Source: CAD feature listing. Evaluate the final solid. Frame: model axes, mm. Give positions to 0.01 mm unless a question says otherwise; leave off trailing zeros. Loops run counter-clockwise (first coordinate to the right, second up) from the corner with the lowest first, then second, coordinate; pieces in that order, holes last. Notation, with made-up numbers: M 77,30.25 L 125,30.25 A17 ccw 125,57.25 Z; hole C -14.5,34 d5. An arc over 180 degrees is marked long. Answer in a Markdown table with one row per item.
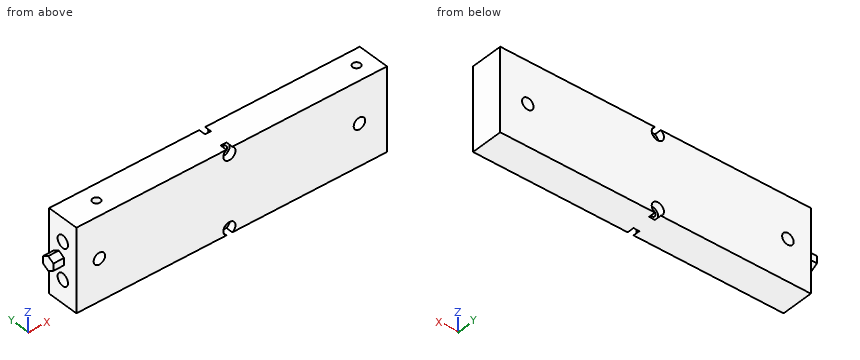
```python
from build123d import *

# Parameters (mm, degrees)
SKETCH_1_W          = 203
SKETCH_1_H          = 54
EXTRUDE_1_DEPTH     = 21
SKETCH_2_R          = 4
CUT_EXTRUDE_1_DEPTH = 150
SKETCH_3_R          = 2.25
CUT_EXTRUDE_2_DEPTH = 212.106608139
SKETCH_4_R          = 4
CUT_EXTRUDE_3_DEPTH = 4.5
SKETCH_5_R          = 3.75
CUT_EXTRUDE_4_DEPTH = 7.2
SKETCH_6_R          = 2.5
CUT_EXTRUDE_5_DEPTH = 5
EXTRUDE_2_DEPTH     = 7


with BuildPart() as part:
    # 草图1 → 凸台-拉伸1 (new body)
    with BuildSketch(Plane(origin=(0, 0, 0), x_dir=(1, 0, 0), z_dir=(0, 1, 0))):
        with Locations((101.5, 27)):
            Rectangle(SKETCH_1_W, SKETCH_1_H)
    extrude(amount=EXTRUDE_1_DEPTH)

    # 草图2 → 切除-拉伸1 (cut)
    with BuildSketch(Plane.ZY):
        with Locations((-15, 10.5)):
            Circle(SKETCH_2_R)
        with Locations(Location((-39, 10.5, 0), (0, 0, 180))):
            Circle(SKETCH_2_R)
    extrude(amount=-CUT_EXTRUDE_1_DEPTH, mode=Mode.SUBTRACT)

    # 草图3 → 切除-拉伸2 (cut, through all)
    with BuildSketch(Plane(origin=(0, 21, 0), x_dir=(1, 0, 0), z_dir=(0, 1, 0))):
        with Locations(Location((100, 3.5, 0), (0, 0, 270))):
            Circle(SKETCH_3_R)
        with Locations(Location((100, 50.5, 0), (0, 0, 270))):
            Circle(SKETCH_3_R)
        with Locations(Location((15, 27, 0), (0, 0, 270))):
            Circle(SKETCH_3_R)
        with Locations(Location((185, 27, 0), (0, 0, 270))):
            Circle(SKETCH_3_R)
    extrude(amount=-CUT_EXTRUDE_2_DEPTH, mode=Mode.SUBTRACT)

    # 草图4 → 切除-拉伸3 (cut)
    with BuildSketch(Plane(origin=(0, 21, 0), x_dir=(1, 0, 0), z_dir=(0, 1, 0))):
        with Locations((100, 50.5)):
            Circle(SKETCH_4_R)
        with Locations((100, 3.5)):
            Circle(SKETCH_4_R)
    cut_extrude_3 = extrude(amount=-CUT_EXTRUDE_3_DEPTH, mode=Mode.SUBTRACT)

    # 草图5 → 切除-拉伸4 (cut)
    with BuildSketch(Plane(origin=(0, 21, 0), x_dir=(1, 0, 0), z_dir=(0, 1, 0))):
        with Locations(Location((185, 27, 0), (0, 0, 270))):
            Circle(SKETCH_5_R)
        with Locations(Location((15, 27, 0), (0, 0, 270))):
            Circle(SKETCH_5_R)
    cut_extrude_4 = extrude(amount=-CUT_EXTRUDE_4_DEPTH, mode=Mode.SUBTRACT)

    # 镜向1: 切除-拉伸3, 切除-拉伸4 across plane
    add(cut_extrude_3.mirror(Plane(origin=(0, 10.5, 0), x_dir=(0, 0, 1), z_dir=(0, -1, 0))), mode=Mode.SUBTRACT)
    add(cut_extrude_4.mirror(Plane(origin=(0, 10.5, 0), x_dir=(0, 0, 1), z_dir=(0, -1, 0))), mode=Mode.SUBTRACT)

    # 草图6 → 切除-拉伸5 (cut)
    with BuildSketch(Plane.XY):
        with Locations((22, 10.5)):
            Circle(SKETCH_6_R)
        with Locations((192, 10.5)):
            Circle(SKETCH_6_R)
    extrude(amount=-CUT_EXTRUDE_5_DEPTH, mode=Mode.SUBTRACT)

    # 草图7 → 凸台-拉伸2 (add)
    with BuildSketch(Plane.ZY):
        Polygon((-24.690598923, 17.5), (-29.309401077, 17.5), (-31.618802154, 13.5), (-29.309401077, 9.5), (-24.690598923, 9.5), (-22.381197846, 13.5), align=None)
    extrude(amount=EXTRUDE_2_DEPTH)


solid = part.part
```
1) Section C-C, the plane z = -39. Return loops of the section in (x, y), then the cut area to 3 significant figures.
Reply:
| item | result |
|---|---|
| outline | M 0,0 L 203,0 L 203,21 L 0,21 L 0,14.5 L 150,14.5 L 150,6.5 L 0,6.5 Z |
| area | 3,060 mm² |
2) Material intervals for L1, parallel to Y at x = 57, z = -15; L2, parallel to X at y = 3.25, z = -29; L3, parallel to Y at x = 97, z = -51.5, sorted ascending.
Reply:
| item | result |
|---|---|
| L1 | y = 0 to 6.5, 14.5 to 21 |
| L2 | x = 0 to 11.83, 18.17 to 181.83, 188.17 to 203 |
| L3 | y = 4.5 to 16.5 |
3) Pin query (flat end, axial travel): pin 1 Ø12 at (x, z) = (185, -27) entering from -Y; pin 2 Ø2 at (x, z) = (98, -49.5) entering from -Y; pin 3 Ø4 at (x, z) = (186, -27) entering from +Y; pin 4 Ø4 at (y, z) = (12.5, -39.5) entering from -X. Return the tip coordinate at first contact, or that it passes through.
Reply:
| item | result |
|---|---|
| pin 1 | stops at y = 0 |
| pin 2 | stops at y = 4.5 |
| pin 3 | stops at y = 13.8 |
| pin 4 | stops at x = 0 |
4) Section D-D, the plane x = 50.5. Return loops of the section in (y, z).
Reply:
| item | result |
|---|---|
| outline | M 0,-54 L 21,-54 L 21,0 L 0,0 Z; hole C 10.5,-39 d8; hole C 10.5,-15 d8 |
5) Section A-A, the plane x = 100. Return loops of the section in (y, z), then the cut area to 3 significant figures.
Reply:
| item | result |
|---|---|
| outline | M 0,-46.5 L 4.5,-46.5 L 4.5,-48.25 L 16.5,-48.25 L 16.5,-46.5 L 21,-46.5 L 21,-7.5 L 16.5,-7.5 L 16.5,-5.75 L 4.5,-5.75 L 4.5,-7.5 L 0,-7.5 Z; M 4.5,-54 L 16.5,-54 L 16.5,-52.75 L 4.5,-52.75 Z; M 4.5,-1.25 L 16.5,-1.25 L 16.5,0 L 4.5,0 Z; hole C 10.5,-39 d8; hole C 10.5,-15 d8 |
| area | 790 mm² |
6) Section B-B, the plane x = 22. Return loops of the section in (y, z).
Reply:
| item | result |
|---|---|
| outline | M 0,-54 L 21,-54 L 21,0 L 13,0 L 13,-5 L 8,-5 L 8,0 L 0,0 Z; hole C 10.5,-39 d8; hole C 10.5,-15 d8 |
